Model file for the job. Use its own axes, mm. A direction names the side the tool comes from. Round coordinates to 2 decimals unless told otherwise and drop trailing zeros. Write each loop counter-clockwise with the first axis right and the second up, starting at its lowest first coordinate (ties: lowest second). Pieces come first, ordered by that corner, then holes. Notation, with made-up numbers: (-19, 57.25) - (19, 57.25) arc R24 ccw to (19, 67.25) - close; hole circle Ø7 at (-7, 61.5). An arc over 180 degrees is marked (long way). One line per item, written item: value.
from build123d import *

# Parameters (mm, degrees)
SKETCH_1_W          = 20
SKETCH_1_H          = 20
SKETCH_1_W_2        = 17
SKETCH_1_H_2        = 17
EXTRUDE_1_DEPTH     = 185
SKETCH_2_R          = 2.05
CUT_EXTRUDE_1_DEPTH = 187.346451536
SKETCH_3_R          = 2
CUT_EXTRUDE_2_DEPTH = 187.346451536
SKETCH_4_R          = 3
CUT_EXTRUDE_3_DEPTH = 187.346451536


with BuildPart() as part:
    # 草图1 → 凸台-拉伸1 (new body)
    with BuildSketch(Plane.XY):
        Rectangle(SKETCH_1_W, SKETCH_1_H)
        Rectangle(SKETCH_1_W_2, SKETCH_1_H_2, mode=Mode.SUBTRACT)
    extrude(amount=EXTRUDE_1_DEPTH)

    # 草图2 → 切除-拉伸1 (cut, through all)
    with BuildSketch(Plane(origin=(0, 10, 0), x_dir=(1, 0, 0), z_dir=(0, 1, 0))):
        with Locations(Location((0, -180, 0), (0, 0, 270))):
            Circle(SKETCH_2_R)
        with Locations(Location((0, -165, 0), (0, 0, 270))):
            Circle(SKETCH_2_R)
    extrude(amount=-CUT_EXTRUDE_1_DEPTH, mode=Mode.SUBTRACT)

    # 草图3 → 切除-拉伸2 (cut, through all)
    with BuildSketch(Plane(origin=(10, 0, 0), x_dir=(0, 0, -1), z_dir=(1, 0, 0))):
        with Locations(Location((-25, 0, 0), (0, 0, 90))):
            Circle(SKETCH_3_R)
        with Locations(Location((-40, 0, 0), (0, 0, 90))):
            Circle(SKETCH_3_R)
    extrude(amount=-CUT_EXTRUDE_2_DEPTH, mode=Mode.SUBTRACT)

    # 草图4 → 切除-拉伸3 (cut, through all)
    with BuildSketch(Plane.ZY.offset(10)):
        with Locations((60, 0)):
            Circle(SKETCH_4_R)
    extrude(amount=-CUT_EXTRUDE_3_DEPTH, mode=Mode.SUBTRACT)


solid = part.part
1. Band-saw the part on D-D on z = 112. Write the cut outline in (x, y).
Report:
outline: (-10, -10) - (10, -10) - (10, 10) - (-10, 10) - close; hole (-8.5, -8.5) - (8.5, -8.5) - (8.5, 8.5) - (-8.5, 8.5) - close
2. Mould opens along Z. For faces 3 (the face through (-9, 0, 185)), 4 (the face through (-8.5, 0, 91)), 5 (the face through (-9, 0, 38)) say: released by +Z, released by -Z, zero draft, split by the parting line, or undercut.
Report:
face 3: released by +Z
face 4: zero draft
face 5: undercut
3. Wall check: probe 1 along Y at (x, z) = (-5.5, 114.5); probe 2 along X at (y, z) = (-9.55, 180). Give the ranges that are in metal, low to high. Write a range as [from, to].
Report:
probe 1: [-10, -8.5], [8.5, 10]
probe 2: [-10, -2.05], [2.05, 10]
4. Band-saw the part on A-A on y = 6. Write the cut outline in (x, z), plus the area to 3 significant figures.
Report:
outline: (-10, 0) - (-8.5, 0) - (-8.5, 185) - (-10, 185) - close; (8.5, 0) - (10, 0) - (10, 185) - (8.5, 185) - close
area: 555 mm²
5. Tool access for faces 1 (the face through (9, 0, 23)), 2 (the face through (8.5, 0, 91)): list every direction of +Z, -Z, +X, -X, +Y, -Y with a clear straight run to the whole face (end or side of a thin tool).
Report:
face 1: +X, -X
face 2: +Z, -Z
6. Band-saw the part on B-B on z = 165. Write the cut outline in (x, y).
Report:
outline: (-10, -10) - (-2.05, -10) - (-2.05, -8.5) - (-8.5, -8.5) - (-8.5, 8.5) - (-2.05, 8.5) - (-2.05, 10) - (-10, 10) - close; (2.05, -10) - (10, -10) - (10, 10) - (2.05, 10) - (2.05, 8.5) - (8.5, 8.5) - (8.5, -8.5) - (2.05, -8.5) - close
